from build123d import *

# Parameters (mm, degrees)
SKETCH1_R         = 171.45
EXTRUDE1_DEPTH    = 36.5125
SKETCH2_R         = 11.1125
EXTRUDE2_DEPTH    = 246.20066814
CIRPATTERN1_COUNT = 8
FILLET1_R         = 1.154545455


with BuildPart() as part:
    # Sketch1 → Extrude1 (new body)
    with BuildSketch(Plane.XY):
        Circle(SKETCH1_R)
    extrude(amount=EXTRUDE1_DEPTH)

    # Sketch2 → Extrude2 (cut, through all)
    with BuildSketch(Plane.XY.offset(36.5125)):
        with Locations((0, 149.225)):
            Circle(SKETCH2_R)
    extrude2 = extrude(amount=-EXTRUDE2_DEPTH, mode=Mode.SUBTRACT)

    # CirPattern1: Extrude2 ×8 about axis
    cirpattern1_axis = Axis((0, 0, 0), (0, 0, 1))
    for i in range(1, CIRPATTERN1_COUNT):
        add(extrude2.rotate(cirpattern1_axis, i * 360 / CIRPATTERN1_COUNT), mode=Mode.SUBTRACT)

    # Sketch3 → Cut-Revolve1 (revolve, cut)
    with BuildSketch(Plane(origin=(0, 0, 0), x_dir=(0, 0, -1), z_dir=(1, 0, 0))):
        Polygon((-36.5125, 109.9185), (-18.25625, 109.347), (-18.25625, 0), (-36.5125, 0), align=None)
    revolve(axis=Axis((0, 0, 18.25625), (0, 0, 1)), mode=Mode.SUBTRACT)

    # Fillet1
    fillet1_edges = [part.edges().sort_by_distance(p)[0] for p in [
        (0, -109.347, 18.25625),
        (0, -109.9185, 36.5125),
        (-171.45, 0, 36.5125),
    ]]
    fillet(fillet1_edges, radius=FILLET1_R)


solid = part.part
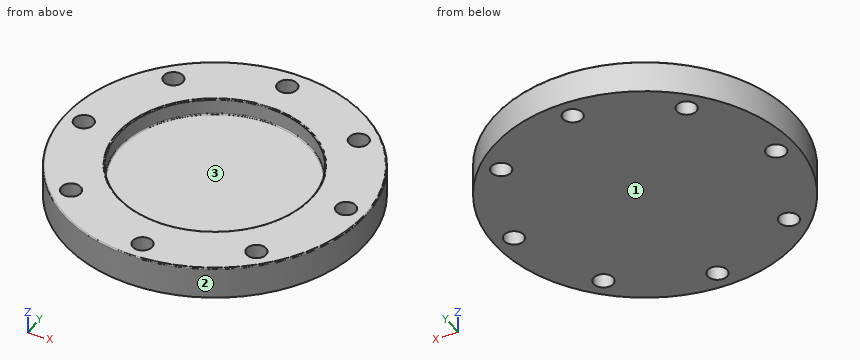
The listing builds one solid part. Answer for the finished solid, in the listing's coordinates (mm). Face numbers are marked on the shaded views. Coordinates: 2 decimals unless noted, no trailing zeros. Loops run counter-clockwise (first coordinate to the right, second up) from the corner with the lowest first, then second, coordinate; pieces in that order, holes last.
1) Find the intervals of material crossed by L1, parallel to Y at x = -1, z = 3; L2, parallel to X at y = -97, z = 33.5; L3, parallel to Y at x = -96.5, z = 12.5, in increasing order.
2) Find section A-A on x = 0. Write down the section's boundary in (y, z), then the cut area to 3 significant figures.
3) Determine the mould class of the marked faces 1, 2 and 3 for opening direction X: pulls with the +X half, pulls with the -X half, needs draft (parallel to the pull), parting line crosses it, or undercut.
4) Flat-ended cylindrical pins translate along their axes: pin 1 Ø20 at (x, y) = (105.52, -105.52) entering from +Z; pin 2 Ø10 at (y, z) = (-128, 26.5) entering from -X; pin 3 Ø10 at (y, z) = (-66.5, 8) entering from -X; pin 4 Ø4 at (x, z) = (90, 10.5) entering from -Y. Find the tip coordinate at first contact, or state that the pin passes through.
5) Find section C-C on z = 10.5. Give the number of separate pieces and of enclosed holes in the cut face, then the cut area to 3 significant figures.
Values:
1. L1: y = -171.45 to -160.29, -138.16 to 138.16, 160.29 to 171.45
1. L2: x = -141.37 to -112.65, -98.38 to -51.5, 51.5 to 98.38, 112.65 to 141.37
1. L3: y = -141.71 to -112.01, -99.02 to 99.02, 112.01 to 141.71
2. outline: (-171.45, 0) - (-160.34, 0) - (-160.34, 36.51) - (-170.3, 36.51) arc R1.15 ccw to (-171.45, 35.36) - close; (-138.11, 0) - (138.11, 0) - (138.11, 36.51) - (111.04, 36.51) arc R1.15 ccw to (109.88, 35.39) - (109.38, 19.37) arc R1.15 cw to (108.23, 18.26) - (-108.23, 18.26) arc R1.15 cw to (-109.38, 19.37) - (-109.88, 35.39) arc R1.15 ccw to (-111.04, 36.51) - (-138.11, 36.51) - close; (160.34, 0) - (171.45, 0) - (171.45, 35.36) arc R1.15 ccw to (170.3, 36.51) - (160.34, 36.51) - close
2. area: 6,890 mm2
3. face 1: needs draft
3. face 2: parting line crosses it
3. face 3: undercut
4. pin 1: passes through
4. pin 2: stops at x = -119.44
4. pin 3: stops at x = -160.04
4. pin 4: stops at y = -147.14
5. separate pieces: 1
5. enclosed holes: 8
5. area: 89,200 mm2
